```python
from build123d import *

# Parameters (mm, degrees)
F1_DEPTH = 12.7
F2_DEPTH = 6.35
F0_W     = 8.346368
F0_H     = 13.526869
F3_DEPTH = 25.4
F4_DEPTH = 50.8
F5_DEPTH = 1.27


with BuildPart() as f1:
    # F0 (on Front) → F1 (new body, symmetric)
    with BuildSketch(Plane.XZ):
        with BuildLine():
            Line((-42.533579, 0), (-23.373938, 0))
            ThreePointArc((-23.373938, 0), (-15.291708, 3.347769), (-11.943938, 11.43))
            Line((-11.943938, 11.43), (-11.943938, 18.357894))
            ThreePointArc((-11.943938, 18.357894), (-15.291708, 26.440125), (-23.373938, 29.787894))
            Line((-23.373938, 29.787894), (-42.533579, 29.787894))
            ThreePointArc((-42.533579, 29.787894), (-50.61581, 26.440125), (-53.963579, 18.357894))
            Line((-53.963579, 18.357894), (-53.963579, 11.43))
            ThreePointArc((-53.963579, 11.43), (-50.61581, 3.347769), (-42.533579, 0))
        make_face()
    extrude(amount=F1_DEPTH, both=True)

    # F0 (on Front) → F2 (join, symmetric)
    with BuildSketch(Plane.XZ):
        with BuildLine():
            ThreePointArc((-11.943938, 11.43), (-15.291708, 3.347769), (-23.373938, 0))
            Line((-23.373938, 0), (-11.943938, 0))
            Line((-11.943938, 0), (43.026961, 29.787894))
            Line((43.026961, 29.787894), (43.026961, 58.54751))
            Line((43.026961, 58.54751), (-11.943938, 29.787894))
            Line((-11.943938, 29.787894), (-23.373938, 29.787894))
            ThreePointArc((-23.373938, 29.787894), (-15.291708, 26.440125), (-11.943938, 18.357894))
            Line((-11.943938, 18.357894), (-11.943938, 11.43))
        make_face()
    extrude(amount=F2_DEPTH, both=True)

    # F0 (on Front) → F3 (join, symmetric)
    with BuildSketch(Plane.XZ):
        Polygon((43.026961, 58.54751), (43.026961, 29.787894), (49.09091, 29.787894), (65.763615, 29.787894), (65.763615, 58.54751), align=None)
        with Locations((54.683095, 44.322086)):
            Rectangle(F0_W, F0_H, mode=Mode.SUBTRACT)
    extrude(amount=F3_DEPTH, both=True)

    # F0 (on Front) → F4 (join, symmetric)
    with BuildSketch(Plane.XZ):
        with Locations((54.683095, 44.322086)):
            Rectangle(F0_W, F0_H)
    extrude(amount=F4_DEPTH, both=True)

    # F0 (on Front) → F5 (join, symmetric)
    with BuildSketch(Plane.XZ):
        with BuildLine():
            Line((-11.943938, 0), (-23.373938, 0))
            Line((-23.373938, 0), (-42.533579, 0))
            ThreePointArc((-42.533579, 0), (-50.61581, 3.347769), (-53.963579, 11.43))
            Line((-53.963579, 11.43), (-53.963579, 18.357894))
            ThreePointArc((-53.963579, 18.357894), (-50.61581, 26.440125), (-42.533579, 29.787894))
            Line((-42.533579, 29.787894), (-23.373938, 29.787894))
            Line((-23.373938, 29.787894), (-11.943938, 29.787894))
            Line((-11.943938, 29.787894), (43.026961, 58.54751))
            ThreePointArc((43.026961, 58.54751), (-91.839408, 15.091917), (49.09091, 29.787894))
            Line((49.09091, 29.787894), (43.026961, 29.787894))
            Line((43.026961, 29.787894), (-11.943938, 0))
        make_face()
    extrude(amount=F5_DEPTH, both=True)


solid = f1.part
```
Verification items for the finished model (mm, model axes). A direction names the side the tool comes from. Round coordinates to 2 decimals unless told otherwise and drop trailing zeros. Write each loop counter-clockwise with the first axis right and the second up, starting at its lowest first coordinate (ties: lowest second). Pieces come first, ordered by that corner, then holes. Notation, with made-up numbers: (-24.75, 7) - (-0.75, 7) arc R30 ccw to (-0.75, 33) - close; hole circle Ø10 at (-5, 51). An arc over 180 degrees is marked (long way). Answer as a JSON object with one key per item and string values. Group by question number.
Q1. Tool access check on faces 1 (the flat face through (50.51, -38, 44)), 2 (the flat face through (58.856, 38, 44)), 3 (the cylindrical face through (-50.526, -7.065, 26.529)), 4 (the flat face through (58.856, -38, 44)), 5 (the cylindrical face through (-15.38, 9.48, 3.26)). Record the directions out of +Z, -Z, +X, -X, +Y, -Y that give a thin tool (end or side, any length) a straight path to the whole face; none if there is none.
Q2. Section check A-A, the plane x = 15.5. Enter the section's corners in (y, z).
Q3. Section check C-C, the plane y = 35. Enter the section's corners in (x, z), plus the area to 3 significant figures.
Q4. Go/stop test with flat-tipped pins: pin 1 Ø5 at (x, z) = (-15.5, -26.5) entering from -Y; pin 2 Ø15 at (y, z) = (44.5, 46.5) entering from -X; pin 3 Ø15 at (x, z) = (-24, 13) entering from +Y. Record where each tip stops, or that it passes through.
Q5. Thickness scan on line 1 (Y direction, x = 31.5, z = 20); line 2 (X direction, y = -29, z = 39); line 3 (Z direction, x = 55, y = -22). Record the ranges inside material, lowest first.
Q6. Section check B-B, the plane z = 47.5. Enter the section's corners in (x, y), plus the area to 3 significant figures.
Q7. Section check D-D, the plane x = 39.5. Enter the section's corners in (y, z), plus the area to 3 significant figures.
Found:
{
 "1": {"face 1": "+Z, -Z, -X, -Y", "face 2": "+Z, -Z, +X, +Y", "face 3": "+Z, -X, -Y", "face 4": "+Z, -Z, +X, -Y", "face 5": "-Z, +X, +Y"},
 "2": {"outline": "(-6.35, 14.87) - (-1.27, 14.87) - (-1.27, -30.69) - (1.27, -30.69) - (1.27, 14.87) - (6.35, 14.87) - (6.35, 44.15) - (1.27, 44.15) - (1.27, 90.26) - (-1.27, 90.26) - (-1.27, 44.15) - (-6.35, 44.15) - close"},
 "3": {"outline": "(50.51, 37.56) - (58.86, 37.56) - (58.86, 51.09) - (50.51, 51.09) - close", "area": "113 mm^2"},
 "4": {"pin 1": "stops at y = -1.27", "pin 2": "stops at x = 50.51", "pin 3": "stops at y = 12.7"},
 "5": {"line 1": "y = -1.27 to 1.27", "line 2": "x = 50.51 to 58.86", "line 3": "z = 29.79 to 58.55"},
 "6": {"outline": "(-91.13, -1.27) - (21.91, -1.27) - (21.91, -6.35) - (43.03, -6.35) - (43.03, -25.4) - (50.51, -25.4) - (50.51, -50.8) - (58.86, -50.8) - (58.86, -25.4) - (65.76, -25.4) - (65.76, 25.4) - (58.86, 25.4) - (58.86, 50.8) - (50.51, 50.8) - (50.51, 25.4) - (43.03, 25.4) - (43.03, 6.35) - (21.91, 6.35) - (21.91, 1.27) - (-91.13, 1.27) - close", "area": "2,130 mm^2"},
 "7": {"outline": "(-6.35, 27.88) - (-1.27, 27.88) - (-1.27, -5.91) - (1.27, -5.91) - (1.27, 27.88) - (6.35, 27.88) - (6.35, 56.7) - (1.27, 56.7) - (1.27, 65.49) - (-1.27, 65.49) - (-1.27, 56.7) - (-6.35, 56.7) - close", "area": "474 mm^2"}
}
